```python
from build123d import *

# Parameters (mm, degrees)
SKETCH3_W          = 10
SKETCH3_H          = 3
SKETCH5_R          = 1.5
CUT_EXTRUDE2_DEPTH = 57.489403968
SKETCH2_R          = 2.032
CUT_EXTRUDE1_DEPTH = 56.009569719
FILLET1_R          = 5


with BuildPart() as part:
    # Sweep1: sweep along a path in Sketch4
    with BuildLine(Plane.XY) as sweep1_path:
        Line((-45.175097276, 1.5), (-25.175097276, 1.5))
        ThreePointArc((-25.175097276, 1.5), (-22.696809318, 1.811961561), (-20.373147477, 2.72838224))
        Line((-20.373147477, 2.72838224), (22.632771246, 26.27161776))
        ThreePointArc((22.632771246, 26.27161776), (24.956433088, 27.188038439), (27.434721046, 27.5))
        Line((27.434721046, 27.5), (47.434721046, 27.5))
    # Sketch3 → Sweep1 (sweep)
    with BuildSketch(Plane.ZY.offset(45.175097276)):
        with Locations((5, 0)):
            Rectangle(SKETCH3_W, SKETCH3_H)
    sweep(path=sweep1_path.line)

    # Sketch5 → Cut-Extrude2 (cut, through all)
    with BuildSketch(Plane(origin=(0, 27.5, 0), x_dir=(1, 0, 0), z_dir=(0, 1, 0))):
        with Locations(Location((43.434721046, -5, 0), (0, 0, 180))):
            Circle(SKETCH5_R)
    extrude(amount=-CUT_EXTRUDE2_DEPTH, mode=Mode.SUBTRACT)

    # Sketch2 → Cut-Extrude1 (cut, through all)
    with BuildSketch(Plane(origin=(0, 1.5, 0), x_dir=(1, 0, 0), z_dir=(0, 1, 0))):
        with Locations(Location((-40.175097276, -5, 0), (0, 0, 270))):
            Circle(SKETCH2_R)
    extrude(amount=-CUT_EXTRUDE1_DEPTH, mode=Mode.SUBTRACT)

    # Fillet1
    fillet1_edges = [part.edges().sort_by_distance(p)[0] for p in [
        (47.434721046, 26, 0),
        (47.434721046, 26, 10),
        (-45.175097276, 0, 10),
        (-45.175097276, 0, 0),
    ]]
    fillet(fillet1_edges, radius=FILLET1_R - 0.0001)  # a hair under: the kernel refuses the full size


solid = part.part
```
Input: part model. Units: mm. Frame: model coordinates. A direction names the side the tool comes from. Coordinates: 2 decimals unless noted, no trailing zeros. Loops run counter-clockwise (first coordinate to the right, second up) from the corner with the lowest first, then second, coordinate; pieces in that order, holes last. Notation, with made-up numbers: M 20.25,64.25 L 71.25,64.25 A7 ccw 71.25,76.25 Z; hole C -20,5 d1. An arc over 180 degrees is marked long. One line per item, written item: value.
(1) Pin query (flat end, axial travel): pin 1 (4 mm diameter, centred on y = 21, z = 2.5, fed in from +X); pin 2 (3 mm diameter, centred on x = -36, z = 7, fed in from +Y); pin 3 (4 mm diameter, centred on y = 5.5, z = 8, fed in from +X); pin 4 (2.5 mm diameter, centred on x = 43.43, z = 5, fed in from -Y). Return the tip coordinate at first contact, or that it passes through.
Filled in:
pin 1: x = 22.9
pin 2: y = 1.5
pin 3: x = -5.41
pin 4: through
(2) Line query: line 1 along Y through (x, z) = (-26.5, 5.75); line 2 along X through (y, z) = (0.3, 5); line 3 along Y through (x, z) = (41, 2.5). Output: solid intervals per line, ascending. Write a range as from..to.
Filled in:
line 1: -1.5..1.5
line 2: -45.18..-42.21, -38.14..-18.56
line 3: 24.5..27.5
(3) Section A-A (x = 41). Output: boundary loops of the cut face in (y, z).
Filled in:
outline: M 24.5,0 L 27.5,0 L 27.5,10 L 24.5,10 Z
(4) Reachability of faces 1 (the flat face through (-35, -1.5, 5)), 2 (the flat face through (-35, 1.5, 5)) from +Z, -Z, +X, -X, +Y, -Y: full face, straight path, thin tool, end or side. Return the list, or none.
Filled in:
face 1: +Z, -Z, +X, -X, -Y
face 2: +Z, -Z, -X, +Y
(5) Pull-direction query (X, two-part tool) for faces 3 (the cylindrical face through (-21.998, -1.106, 5.07)), 4 (the flat face through (38, 24.5, 5)), 5 (the flat face through (1.431, 14.665, 5.07)), 6 (the cylindrical face through (44.933, 26.021, 5.066)); classes: +X half, -X half, draft (parallel to the pull), parting line (faces both ways), or undercut.
Filled in:
face 3: +X half
face 4: draft
face 5: -X half
face 6: undercut
(6) Section B-B (y = 18.5). Output: boundary loops of the cut face in (x, z), and give its area (3 significant figures).
Filled in:
outline: M 8.44,0 L 14.68,0 L 14.68,10 L 8.44,10 Z
area: 62.5 mm^2
